Autodesk Inventor part; units mm, degrees
ref_plane "YZ Plane" through (0, 0, 0) normal (1, 0, 0) x (0, 1, 0)
ref_plane "XZ Plane" through (0, 0, 0) normal (0, 1, 0) x (-1, 0, 0)
ref_plane "XY Plane" through (0, 0, 0) normal (0, 0, 1) x (1, 0, 0)
sketch "Boceto1" plane through (0, 0, 0) normal (0, 0, 1) x (1, 0, 0)
  line L0 (-55, 80) -> (55, 80)
  line L1 (55, 80) -> (55, -80)
  line L2 (55, -80) -> (-55, -80)
  line L3 (-55, -80) -> (-55, 80)
  line L4 (-55, 80) -> (55, -80) construction
  line L5 (55, 80) -> (-55, -80) construction
  point P0 (0, 0)
  dimension "d0" = 110
  dimension "d1" = 160
extrude "Placa1" add sketch "Boceto1" along normal blind 0.5
sketch "Boceto2" plane through (0, 0, 0.5) normal (0, 0, 1) x (1, 0, 0)
  line L0 (-38.3122, 60.4154) -> (41.6878, 60.4154)
  line L1 (41.6878, 60.4154) -> (41.6878, 20.4154)
  line L2 (41.6878, 20.4154) -> (-38.3122, 20.4154)
  line L3 (-38.3122, 20.4154) -> (-38.3122, 60.4154)
  line L4 (-26.0335, -16.1653) -> (-26.0335, -22.1653)
  line L5 (-26.0335, -22.1653) -> (-20.0335, -22.1653)
  line L6 (-20.0335, -22.1653) -> (-20.0335, -16.1653)
  line L7 (-20.0335, -16.1653) -> (-26.0335, -16.1653)
  line L8 (-16.6334, -22.1653) -> (-16.6334, -16.1653)
  line L9 (-16.6334, -16.1653) -> (-10.6334, -16.1653)
  line L10 (-10.6334, -16.1653) -> (-10.6334, -22.1653)
  line L11 (-10.6334, -22.1653) -> (-16.6334, -22.1653)
  line L12 (-7.6728, -22.1653) -> (-7.6728, -16.1653)
  line L13 (-7.6728, -16.1653) -> (-1.6728, -16.1653)
  line L14 (-1.6728, -16.1653) -> (-1.6728, -22.1653)
  line L15 (-1.6728, -22.1653) -> (-7.6728, -22.1653)
  line L16 (1.6878, -22.1653) -> (1.6878, -16.1653)
  line L17 (1.6878, -16.1653) -> (7.6878, -16.1653)
  line L18 (7.6878, -16.1653) -> (7.6878, -22.1653)
  line L19 (7.6878, -22.1653) -> (1.6878, -22.1653)
  line L20 (10.0278, -16.1653) -> (10.0278, -22.1653)
  line L21 (10.0278, -22.1653) -> (16.0278, -22.1653)
  line L22 (16.0278, -22.1653) -> (16.0278, -16.1653)
  line L23 (16.0278, -16.1653) -> (10.0278, -16.1653)
  line L24 (18.758, -22.1653) -> (18.758, -16.1653)
  line L25 (18.758, -16.1653) -> (24.758, -16.1653)
  line L26 (24.758, -16.1653) -> (24.758, -22.1653)
  line L27 (24.758, -22.1653) -> (18.758, -22.1653)
  line L28 (-26.0335, -24.8985) -> (-26.0335, -30.8985)
  line L29 (-26.0335, -30.8985) -> (-20.0335, -30.8985)
  line L30 (-20.0335, -30.8985) -> (-20.0335, -24.8985)
  line L31 (-20.0335, -24.8985) -> (-26.0335, -24.8985)
  line L32 (-16.6334, -24.8985) -> (-16.6334, -30.8985)
  line L33 (-16.6334, -30.8985) -> (-10.6334, -30.8985)
  line L34 (-10.6334, -30.8985) -> (-10.6334, -24.8985)
  line L35 (-10.6334, -24.8985) -> (-16.6334, -24.8985)
  line L36 (-7.6728, -24.8985) -> (-7.6728, -30.8985)
  line L37 (-7.6728, -30.8985) -> (-1.6728, -30.8985)
  line L38 (-1.6728, -30.8985) -> (-1.6728, -24.8985)
  line L39 (-1.6728, -24.8985) -> (-7.6728, -24.8985)
  line L40 (1.6878, -24.8985) -> (1.6878, -30.8985)
  line L41 (1.6878, -30.8985) -> (7.6878, -30.8985)
  line L42 (7.6878, -30.8985) -> (7.6878, -24.8985)
  line L43 (7.6878, -24.8985) -> (1.6878, -24.8985)
  line L44 (16.0278, -24.8985) -> (16.0278, -30.8985)
  line L45 (10.0278, -30.8985) -> (10.0278, -24.8985)
  line L46 (16.0278, -24.8985) -> (10.0278, -24.8985)
  line L47 (10.0278, -30.8985) -> (16.0278, -30.8985)
  line L48 (18.758, -24.8985) -> (18.758, -30.8985)
  line L49 (18.758, -30.8985) -> (24.758, -30.8985)
  line L50 (24.758, -30.8985) -> (24.758, -24.8985)
  line L51 (24.758, -24.8985) -> (18.758, -24.8985)
  point P0 (0, 0)
extrude "Extrusión1" cut sketch "Boceto2" against normal blind 10
sketch "Boceto3" plane through (0, 0, 0.5) normal (0, 0, 1) x (1, 0, 0)
  line L0 (-30.451, -13.5858) -> (-30.451, -33.7304)
  line L1 (-30.451, -33.7304) -> (28.8113, -33.7304)
  line L2 (28.8113, -33.7304) -> (28.8113, -13.5858)
  line L3 (28.8113, -13.5858) -> (-30.451, -13.5858)
  point P0 (0, 0)
extrude "Extrusión2" cut sketch "Boceto3" against normal blind 0.2
equation "\"d2\" = Grosor"
equation "\"Radio_pliegue\" = Grosor"
equation "\"Anchura_desahogo_plegado\" = Grosor"
equation "\"Profundidad_desahogo_plegado\" = 0.5 * Grosor"
equation "\"Tamaño_destalonado\" = 4 * Grosor"
equation "\"Remanente_mínimo\" = 2 * Grosor"
equation "\"Radiodetransición\" = Radio_pliegue"
equation "\"Tamaño_de_radio_de_Jacobi\" = Radio_pliegue"
equation "\"TamañoSeparación\" = Grosor"
properties material "Plástico LCP"
The listing builds one solid part. Answer for the finished solid, in the listing's coordinates (mm). A direction names the side the tool comes from. Give positions to 0.01 mm unless a question says otherwise; leave off trailing zeros. Write each loop counter-clockwise with the first axis right and the second up, starting at its lowest first coordinate (ties: lowest second). Pieces come first, ordered by that corner, then holes.
1) Find the intervals of material crossed by L1, parallel to Y at x = -20.5, z = 0.35; L2, parallel to X at y = 31.5, z = 0.35; L3, parallel to Y at x = -29.5, z = 0.1, in increasing order.
2) A tool of negligible diameter and unlimited length cuts with its end or side. For faces 1 (the face through (-1, -24, 0.3)), 2 (the face through (-1, 1, 0.5)), from which of +Z, -Z, +X, -X, +Y, -Y can it reach the whole face along a straight path? Write none if from no direction.
3) Section A-A (x = 12.5) is taken. Write down the section's boundary in (y, z), and give its area (3 significant figures).
4) Section D-D (x = -32.5) is taken. Write down the section's boundary in (y, z).
5) Section C-C (z = 0.4) is taken. Write down the section's boundary in (x, y).
6) Section B-B (y = 49.5) is taken. Write down the section's boundary in (x, z), and give its area (3 significant figures).
Response:
1. L1: y = -80 to -33.73, -13.59 to 20.42, 60.42 to 80
1. L2: x = -55 to -38.31, 41.69 to 55
1. L3: y = -80 to 20.42, 60.42 to 80
2. face 1: +Z
2. face 2: +Z, +X, -X, +Y, -Y
3. outline: (-80, 0) - (-30.9, 0) - (-30.9, 0.3) - (-33.73, 0.3) - (-33.73, 0.5) - (-80, 0.5) - close; (-24.9, 0) - (-22.17, 0) - (-22.17, 0.3) - (-24.9, 0.3) - close; (-16.17, 0) - (20.42, 0) - (20.42, 0.5) - (-13.59, 0.5) - (-13.59, 0.3) - (-16.17, 0.3) - close; (60.42, 0) - (80, 0) - (80, 0.5) - (60.42, 0.5) - close
3. area: 52.4 mm2
4. outline: (-80, 0) - (20.42, 0) - (20.42, 0.5) - (-80, 0.5) - close; (60.42, 0) - (80, 0) - (80, 0.5) - (60.42, 0.5) - close
5. outline: (-55, -80) - (55, -80) - (55, 80) - (-55, 80) - close; hole (-38.31, 20.42) - (41.69, 20.42) - (41.69, 60.42) - (-38.31, 60.42) - close; hole (-30.45, -33.73) - (28.81, -33.73) - (28.81, -13.59) - (-30.45, -13.59) - close
6. outline: (-55, 0) - (-38.31, 0) - (-38.31, 0.5) - (-55, 0.5) - close; (41.69, 0) - (55, 0) - (55, 0.5) - (41.69, 0.5) - close
6. area: 15.0 mm2
